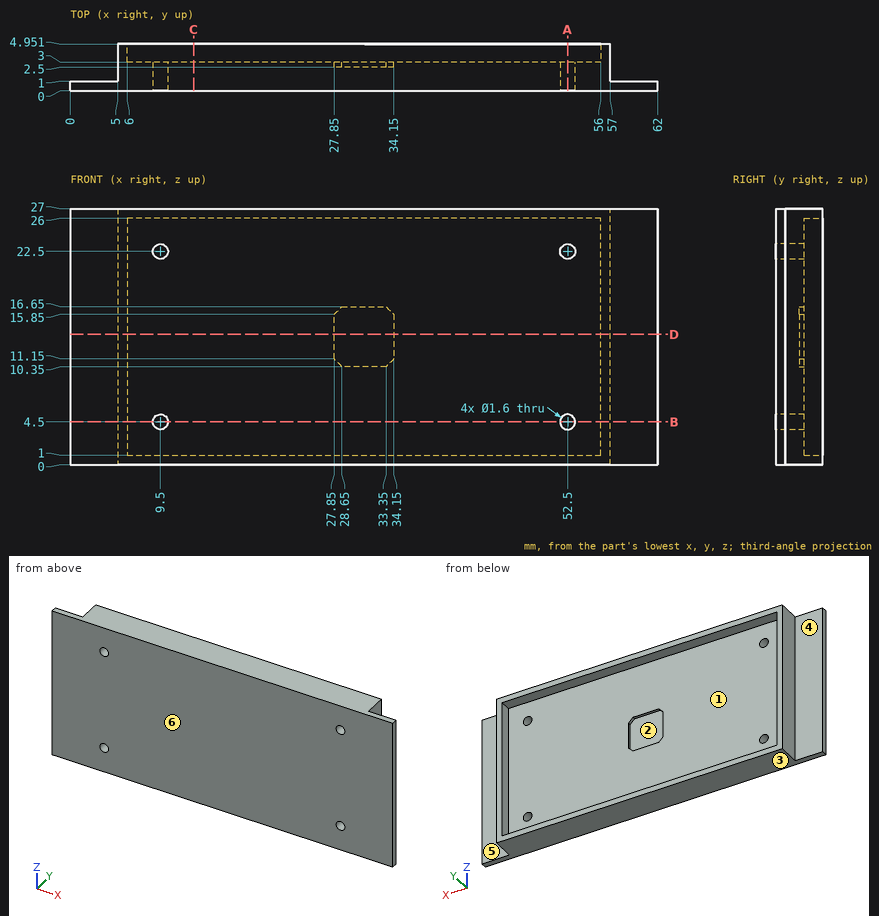
Check sheet for the drawn part. Datum: minimum x, y, z corner. Units: mm. A direction names the side the tool comes from. Coordinates: 2 decimals unless noted, no trailing zeros. Order: outer loops, then holes, each group sorted by start corner. A loop starts at its lowest first (then second) coordinate and runs counter-clockwise, first axis right, second up. Notation, with made-up numbers: M 11.25,85 L 23.25,85 A17 cw 23.25,95 Z; hole C 84.5,54.25 d1. An arc over 180 degrees is marked long. One line per question, with ' | ' between items. Start each with the question number.
Item 1: Cross-section at B-B on z = 4.5. Enter the section's corners in (x, y), then the cut area to 3 significant figures.
Item 2: Cross-section at C-C on x = 13. Enter the section's corners in (y, z), then the cut area to 3 significant figures.
Item 3: Cross-section at D-D on z = 13.75. Enter the section's corners in (x, y), then the cut area to 3 significant figures.
Item 4: Set-up check for the marked faces 5 and 6: record each of +Z, -Z, +X, -X, +Y, -Y from which the full face is reachable in a straight line by a thin tool's end or side.
Item 5: Material ranges on L1, parallel to X at y = 2.2, z = 22.5; L2, parallel to X at y = 0.95, z = 22.5; L3, parallel to Z at x = 52.5, y = 1.45, recorded low to high. Write a range as [from, to].
Item 6: Draft check along Z on the marked faces 1, 2, 3 and 4. Enter one of: pulls with the +Z half, pulls with the -Z half, needs draft (parallel to the pull), parting line crosses it, or undercut.
Item 7: Cross-section at A-A on x = 52.5. Enter the section's corners in (y, z).
Item 8: Gauge pin test, flat ends, axial feed: pin 1 (2.5 mm diameter, centred on x = 52.5, z = 22.5, fed in from +Y); pin 2 (5 mm diameter, centred on x = 54.5, z = 12, fed in from +Y); pin 3 (2 mm diameter, centred on y = 4.5, z = 9.5, fed in from +X); pin 4 (1.4 mm diameter, centred on x = 9.5, z = 4.5, fed in from -Y). Record the tip position at first contact, or that the pin passes through.
Findings:
1) outline: M 0,0 L 8.7,0 L 8.7,3 L 6,3 L 6,4.95 L 5,4.95 L 5,1 L 0,1 Z; M 10.3,0 L 51.7,0 L 51.7,3 L 10.3,3 Z; M 53.3,0 L 62,0 L 62,1 L 57,1 L 57,4.95 L 56,4.95 L 56,3 L 53.3,3 Z | area: 160 mm²
2) outline: M 0,0 L 4.95,0 L 4.95,1 L 3,1 L 3,26 L 4.95,26 L 4.95,27 L 0,27 Z | area: 84.9 mm²
3) outline: M 0,0 L 62,0 L 62,1 L 57,1 L 57,4.95 L 56,4.95 L 56,3 L 34.15,3 L 34.15,2.5 L 27.85,2.5 L 27.85,3 L 6,3 L 6,4.95 L 5,4.95 L 5,1 L 0,1 Z | area: 167 mm²
4) face 5: +Z, -Z, +X, +Y | face 6: +Z, -Z, +X, -X, -Y
5) L1: x = [5, 8.7], [10.3, 51.7], [53.3, 57] | L2: x = [0, 8.7], [10.3, 51.7], [53.3, 62] | L3: z = [0, 3.7], [5.3, 21.7], [23.3, 27]
6) face 1: undercut | face 2: undercut | face 3: pulls with the -Z half | face 4: needs draft
7) outline: M 0,0 L 4.95,0 L 4.95,1 L 3,1 L 3,3.7 L 0,3.7 Z; M 0,5.3 L 3,5.3 L 3,21.7 L 0,21.7 Z; M 0,23.3 L 3,23.3 L 3,26 L 4.95,26 L 4.95,27 L 0,27 Z
8) pin 1: stops at y = 3 | pin 2: stops at y = 4.95 | pin 3: stops at x = 57 | pin 4: passes through
